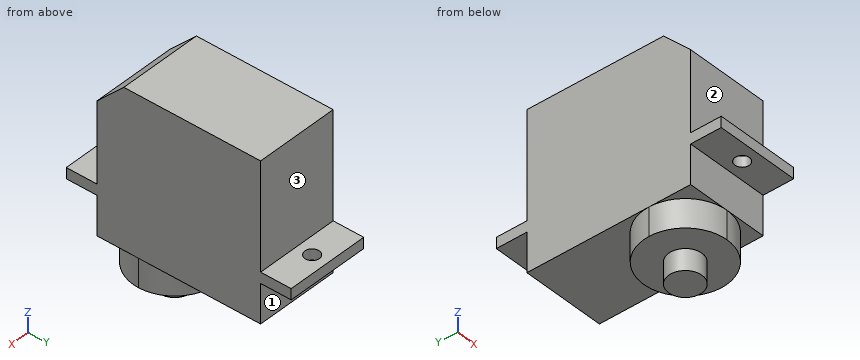
from build123d import *

# Parameters (mm, degrees)
F1_DEPTH = 11.7348
F3_DEPTH = 3.9878
F4_R     = 2.33426
F5_DEPTH = 2.9718
F6_R     = 1.016
F7_DEPTH = 25.4


with BuildPart() as f1:
    # F0 (on Right) → F1 (new body)
    with BuildSketch(Plane.YZ):
        Polygon((0, -15.0368), (0, 0), (-19.304, 0), (-23.114, -3.81), (-23.114, -15.0368), (-27.432, -15.0368), (-27.432, -16.5608), (-23.114, -16.5608), (-23.114, -22.0472), (0, -22.0472), (0, -16.5608), (4.318, -16.5608), (4.318, -15.0368), align=None)
    extrude(amount=F1_DEPTH)

    # F2 (on face) → F3 (join)
    with BuildSketch(Plane(origin=(0, 0, -22.0472), x_dir=(1, 0, 0), z_dir=(0, 0, -1))):
        with BuildLine():
            ThreePointArc((0, 17.2466), (5.8674, 11.3792), (11.7348, 17.2466))
            ThreePointArc((11.7348, 17.2466), (10.016278, 21.395478), (5.8674, 23.114))
            ThreePointArc((5.8674, 23.114), (1.718522, 21.395478), (0, 17.2466))
        make_face()
    extrude(amount=F3_DEPTH)

    # F4 (on face) → F5 (join)
    with BuildSketch(Plane(origin=(0, 0, -26.035), x_dir=(1, 0, 0), z_dir=(0, 0, -1))):
        with Locations((5.8674, 17.2466)):
            Circle(F4_R)
    extrude(amount=F5_DEPTH)

    # F6 (on face) → F7 (cut)
    with BuildSketch(Plane(origin=(0, 0, -16.5608), x_dir=(1, 0, 0), z_dir=(0, 0, -1))):
        with Locations((5.8674, 25.273)):
            Circle(F6_R)
        with Locations((5.8674, -2.159)):
            Circle(F6_R)
    extrude(amount=-F7_DEPTH, mode=Mode.SUBTRACT)


solid = f1.part
CAD build for the part. Positions are in the model's coordinates, mm. Face numbers are marked on the shaded views. A direction names the side the tool comes from. Round coordinates to 2 decimals unless told otherwise and drop trailing zeros. Loops run counter-clockwise (first coordinate to the right, second up) from the corner with the lowest first, then second, coordinate; pieces in that order, holes last. Notation, with made-up numbers: (-4, 76) - (4, 76) arc R23 cw to (4, 104) - close; hole circle Ø6 at (-30, 53.5). An arc over 180 degrees is marked (long way). Put each result on its own line as item: value.
1. Slice it at D-D on z = -20.5. List the corners of the cut face in (x, y), and give its area (3 significant figures).
Geometry check:
outline: (0, -23.11) - (11.73, -23.11) - (11.73, 0) - (0, 0) - close
area: 271 mm²
2. Wall check: line 1 (Z direction, x = 9, y = -16) (3 decimals); line 2 (Z direction, x = 5.75, y = -1); line 3 (Y direction, x = 9.5, z = -6). Give the ranges that are in metal, low to high.
Geometry check:
line 1: -26.035 to 0
line 2: -22.05 to 0
line 3: -23.11 to 0
3. Slice it at B-B on y = -2. List the corners of the cut face in (x, z).
Geometry check:
outline: (0, -22.05) - (11.73, -22.05) - (11.73, 0) - (0, 0) - close
4. Pin check, flat tips, straight feed: P1, Ø1.5, axis at x = 4, y = -10.5, coming from the -Z side; P2, Ø2, axis at x = 4, y = 1.5, coming from the +Z side; P3, Ø3.5, axis at x = 4, z = -11, coming from the +Y side. Stop position of each tip, or through.
Geometry check:
P1: z = -22.05
P2: z = -15.04
P3: y = 0
5. 3-axis set-ups, long thin cutter, end or side, ignore diameter. For the marked faces 1, 2 and 3: which of +Z, -Z, +X, -X, +Y, -Y reach the whole face in a straight line?
Geometry check:
face 1: -Z, +X, -X, +Y
face 2: +Z, +X, -X, -Y
face 3: +Z, +X, -X, +Y
6. Slice it at A-A on x = 6.5. Give the number of separate pieces and of enclosed holes in the cut face, and give its area (3 significant figures).
Geometry check:
separate pieces: 3
enclosed holes: 0
area: 571 mm²
7. Slice it at C-C on x = 10.25. List the corners of the cut face in (y, z) (3 decimals), and give its area (3 significant figures).
Geometry check:
outline: (-27.432, -16.561) - (-23.114, -16.561) - (-23.114, -22.047) - (-21.148, -22.047) - (-21.148, -26.035) - (-13.345, -26.035) - (-13.345, -22.047) - (0, -22.047) - (0, -16.561) - (4.318, -16.561) - (4.318, -15.037) - (0, -15.037) - (0, 0) - (-19.304, 0) - (-23.114, -3.81) - (-23.114, -15.037) - (-27.432, -15.037) - close
area: 547 mm²
